from build123d import *

# Parameters (mm, degrees)
F0_W     = 40
F0_H     = 20
F1_DEPTH = 10
F3_W     = 40
F3_H     = 0.5
F4_DEPTH = 30
F6_R     = 1.49999


# Not quite as in the source:
# - a fillet or chamfer is up to 0.001 mm smaller than in the source, because OpenCascade refuses the exact size


with BuildPart() as f1:
    # F0 (on Top) → F1 (new body)
    with BuildSketch(Plane.XY):
        with Locations((20, -10)):
            Rectangle(F0_W, F0_H)
    extrude(amount=F1_DEPTH)

    # F3 (on face) → F4 (join)
    with BuildSketch(Plane.XY.offset(10)):
        with Locations((20, -3.25)):
            Rectangle(F3_W, F3_H)
        with Locations((20, -6.75)):
            Rectangle(F3_W, F3_H)
        with Locations((20, -10.25)):
            Rectangle(F3_W, F3_H)
        with Locations((20, -13.75)):
            Rectangle(F3_W, F3_H)
        with Locations((20, -17.25)):
            Rectangle(F3_W, F3_H)
    extrude(amount=F4_DEPTH)

    # F5: F1 across face


with BuildPart() as f1_1:
    add(f1.part)
    add(f1.part.mirror(Plane(origin=(20, -17.25, 40), x_dir=(1, 0, 0), z_dir=(0, 0, 1))))

    # F6 (radius 1.5 in the source; OpenCascade refuses exactly that, so slightly less here)
    f6_edges = [f1_1.edges().sort_by_distance(p)[0] for p in [
        (20, -17, 70),
        (20, -13.5, 70),
        (20, -10, 70),
        (20, -6.5, 70),
        (20, -3, 70),
        (20, -3.5, 70),
        (20, -7, 70),
        (20, -10.5, 70),
        (20, -14, 70),
        (20, -17.5, 70),
        (20, -17.5, 10),
        (20, -14, 10),
        (20, -10.5, 10),
        (20, -7, 10),
        (20, -3.5, 10),
        (20, -17, 10),
        (20, -13.5, 10),
        (20, -10, 10),
        (20, -6.5, 10),
        (20, -3, 10),
    ]]
    fillet(f6_edges, radius=F6_R)


solid = f1_1.part
CAD build for the part. Positions are in the model's coordinates, mm. A direction names the side the tool comes from. Round coordinates to 2 decimals unless told otherwise and drop trailing zeros. Loops run counter-clockwise (first coordinate to the right, second up) from the corner with the lowest first, then second, coordinate; pieces in that order, holes last.
(1) Cut at A-A (z = 66). Give the cut face in (x, y), plus the area to 3 significant figures.
(2) Cut at B-B (y = -18.25). Give the cut face in (x, z).
(3) Wall check: line 1 along Y through (x, z) = (7, 32); line 2 along Z through (x, y) = (30, -5); line 3 along Z through (x, y) = (29, -16). Give the ranges that are in metal, low to high.
(4) Cut at C-C (x = 32). State how many separate pieces and enclosed holes the cut face has, plus the area to 3 significant figures.
(5) Which spindle directions (+Z, -Z, +X, -X, +Y, -Y) get a long thin tool onto all of the face, cutting with end or side? Do faces 1 (the cylindrical face through (20.28, -17.93, 69.55)), 2 (the flat face through (20, -7, 40)), 3 (the cylindrical face through (20.28, -2.57, 10.45)). Say none if no direction does.
(6) Drop flat-ended pins along their axis: pin 1 (12 mm diameter, centred on x = 29, z = 28, fed in from +Y); pin 2 (20 mm diameter, centred on x = 12, z = 44, fed in from -Y). Give the stop position or say it passes through.
(7) Two-plate mould, pull along Y, no slides. Class faces 4 (the cylindrical face through (20.28, -7.45, 10.43)), 5 (the flat face through (20, -10, 0)), 6 (the flat face through (20, -3, 40)), 7 (the cylindrical face through (20.28, -7.43, 69.55)): +Y half, -Y half, draft (parallel to the pull), parting line (faces both ways), or undercut.
Findings below:
1. outline: (0, -17.5) - (40, -17.5) - (40, -17) - (0, -17) - close; (0, -14) - (40, -14) - (40, -13.5) - (0, -13.5) - close; (0, -10.5) - (40, -10.5) - (40, -10) - (0, -10) - close; (0, -7) - (40, -7) - (40, -6.5) - (0, -6.5) - close; (0, -3.5) - (40, -3.5) - (40, -3) - (0, -3) - close
1. area: 100 mm2
2. outline: (0, 0) - (40, 0) - (40, 10.2) - (0, 10.2) - close; (0, 69.8) - (40, 69.8) - (40, 80) - (0, 80) - close
3. line 1: y = -17.5 to -17, -14 to -13.5, -10.5 to -10, -7 to -6.5, -3.5 to -3
3. line 2: z = 0 to 10, 70 to 80
3. line 3: z = 0 to 10.09, 69.91 to 80
4. separate pieces: 1
4. enclosed holes: 4
4. area: 560 mm2
5. face 1: +X, -X, -Y
5. face 2: +X, -X
5. face 3: +X, -X, +Y
6. pin 1: stops at y = -3
6. pin 2: stops at y = -17.5
7. face 4: undercut
7. face 5: draft
7. face 6: +Y half
7. face 7: undercut
